from build123d import *

# Parameters (mm, degrees)
SKETCH094_W        = 71
SKETCH094_H        = 81
PAD055_DEPTH       = 5
SKETCH096_W        = 68
SKETCH096_H        = 1.5
PAD053_DEPTH       = 2
SKETCH097_W        = 64.6
SKETCH097_H        = 77.6
PAD054_DEPTH       = 2
SKETCH098_W        = 50
SKETCH098_H        = 72
POCKET086_DEPTH    = 4
SKETCH095_W        = 7.3
SKETCH095_H        = 10
PAD057_DEPTH       = 9
SKETCH099_W        = 5
SKETCH099_H        = 3.5
PAD056_DEPTH       = 9
CHAMFER028_SIZE    = 4.9
SKETCH100_R        = 2.5
POCKET087_DEPTH    = 10
SKETCH102_R        = 2.5
POCKET091_DEPTH    = 10
SKETCH101_R        = 4.5
POCKET088_DEPTH    = 3
POCKET088_FACE29_W = 64.6
POCKET088_FACE29_H = 2
POCKET089_DEPTH    = 2
POCKET089_FACE16_W = 50
POCKET089_FACE16_H = 4
PAD059_DEPTH       = 2
POCKET092_DEPTH    = 2
CHAMFER027_SIZE    = 3
CHAMFER026_SIZE    = 2
SKETCH103_W        = 50
SKETCH103_H        = 72
PAD058_DEPTH       = 2
PAD058_FACE37_W    = 0.5
PAD058_FACE37_H    = 50
POCKET090_DEPTH    = 0.5
PAD061_DEPTH       = 0.5
PAD060_DEPTH       = 0.5
POCKET093_DEPTH    = 1
CHAMFER029_SIZE    = 0.999
FILLET010_R        = 3
POCKET094_DEPTH    = 50


with BuildPart() as part:
    # Sketch094 → Pad055 (new body)
    with BuildSketch(Plane.XY):
        with Locations((-0.121221, -9.466726)):
            Rectangle(SKETCH094_W, SKETCH094_H)
    extrude(amount=-PAD055_DEPTH)

    # Sketch096 (on Face1 of Pad055) → Pad053 (join)
    with BuildSketch(Plane(origin=(0, 31.033274, 0), x_dir=(-1, 0, 0), z_dir=(0, 1, 0))):
        with Locations((0.121221, -0.75)):
            Rectangle(SKETCH096_W, SKETCH096_H)
    extrude(amount=PAD053_DEPTH)

    # Sketch097 (on Face10 of Pad053) → Pad054 (join)
    with BuildSketch(Plane.XY):
        with Locations((-0.121221, -5.766726)):
            Rectangle(SKETCH097_W, SKETCH097_H)
    extrude(amount=PAD054_DEPTH)

    # Sketch098 (on Face13 of Pad054) → Pocket086 (cut)
    with BuildSketch(Plane.XY.offset(2)):
        with Locations((-0.121221, -6.466726)):
            Rectangle(SKETCH098_W, SKETCH098_H)
    extrude(amount=-POCKET086_DEPTH, mode=Mode.SUBTRACT)

    # Sketch095 (on Face14 of Pocket086) → Pad057 (join)
    with BuildSketch(Plane.XY.offset(2)):
        with Locations((28.528779, 28.033274)):
            Rectangle(SKETCH095_W, SKETCH095_H)
        with Locations((-28.771221, 28.033274)):
            Rectangle(SKETCH095_W, SKETCH095_H)
    extrude(amount=PAD057_DEPTH)

    # Sketch099 (on Face1 of Pad057) → Pad056 (join)
    with BuildSketch(Plane.XY.offset(2)):
        with Locations((-22.621221, 31.283274)):
            Rectangle(SKETCH099_W, SKETCH099_H)
        with Locations((22.378779, 31.283274)):
            Rectangle(SKETCH099_W, SKETCH099_H)
    extrude(amount=PAD056_DEPTH)

    # Chamfer028
    chamfer028_edges = [part.edges().sort_by_distance(p)[0] for p in [
        (-20.121221, 31.283274, 11),
        (19.878779, 31.283274, 11),
    ]]
    chamfer(chamfer028_edges, length=CHAMFER028_SIZE)

    # Sketch100 (on Face12 of Chamfer028) → Pocket087 (cut)
    with BuildSketch(Plane(origin=(0, 33.033274, 0), x_dir=(-1, 0, 0), z_dir=(0, 1, 0))):
        with Locations((-28.378779, 6)):
            Circle(SKETCH100_R)
        with Locations((28.621221, 6)):
            Circle(SKETCH100_R)
    extrude(amount=-POCKET087_DEPTH, mode=Mode.SUBTRACT)

    # Sketch102 (on Face30 of Pocket087) → Pocket091 (cut)
    with BuildSketch(Plane(origin=(0, 0, -5), x_dir=(1, 0, 0), z_dir=(0, 0, -1))):
        with Locations((-28.621221, 30.966726)):
            Circle(SKETCH102_R)
        with Locations((28.378779, 30.966726)):
            Circle(SKETCH102_R)
    extrude(amount=-POCKET091_DEPTH, mode=Mode.SUBTRACT)

    # Sketch101 (on Face32 of Pocket091) → Pocket088 (cut)
    with BuildSketch(Plane(origin=(0, 0, -5), x_dir=(1, 0, 0), z_dir=(0, 0, -1))):
        with Locations((-28.621221, 30.966726)):
            Circle(SKETCH101_R)
        with Locations((28.378779, 30.966726)):
            Circle(SKETCH101_R)
    extrude(amount=-POCKET088_DEPTH, mode=Mode.SUBTRACT)

    # Pocket088 Face29 → Pocket089 (cut)
    with BuildSketch(Plane(origin=(-0.121221, -44.566726, 1), x_dir=(-1, 0, 0), z_dir=(0, -1, 0))):
        Rectangle(POCKET088_FACE29_W, POCKET088_FACE29_H)
    extrude(amount=-POCKET089_DEPTH, mode=Mode.SUBTRACT)

    # Pocket089 Face16 → Pad059 (add)
    with BuildSketch(Plane(origin=(-0.121221, -42.466726, 0), x_dir=(1, 0, 0), z_dir=(0, 1, 0))):
        Rectangle(POCKET089_FACE16_W, POCKET089_FACE16_H)
    extrude(amount=PAD059_DEPTH)

    # Pad059 Face1 → Pocket092 (cut)
    with BuildSketch(Plane(origin=(-0.121221, 29.533274, 1.353834), x_dir=(-1, 0, 0), z_dir=(0, -1, 0))):
        Polygon((-25, -9.646166), (-24.9, -9.646166), (-20, -4.746166), (-20, -0.646166), (20, -0.646166), (20, -4.746166), (24.9, -9.646166), (25, -9.646166), (25, 3.353834), (-25, 3.353834), align=None)
    extrude(amount=-POCKET092_DEPTH, mode=Mode.SUBTRACT)

    # Chamfer027
    chamfer027_edges = [part.edges().sort_by_distance(p)[0] for p in [
        (-0.121221, -49.966726, -5),
    ]]
    chamfer(chamfer027_edges, length=CHAMFER027_SIZE)

    # Chamfer026
    chamfer026_edges = [part.edges().sort_by_distance(p)[0] for p in [
        (-28.771221, 23.033274, 11),
        (28.528779, 23.033274, 11),
    ]]
    chamfer(chamfer026_edges, length=CHAMFER026_SIZE)

    # Sketch103 (on Face10 of Chamfer026) → Pad058 (join)
    with BuildSketch(Plane.XY.offset(-2)):
        with Locations((-0.121221, -4.466726)):
            Rectangle(SKETCH103_W, SKETCH103_H)
    extrude(amount=PAD058_DEPTH)

    # Pad058 Face37 → Pocket090 (cut)
    with BuildSketch(Plane(origin=(-0.121221, 31.283274, -2), x_dir=(0, -1, 0), z_dir=(0, 0, -1))):
        Rectangle(PAD058_FACE37_W, PAD058_FACE37_H)
    extrude(amount=-POCKET090_DEPTH, mode=Mode.SUBTRACT)

    # Pocket090 Face9 → Pad061 (add)
    with BuildSketch(Plane(origin=(-32.421221, 7.336396, 2.99136), x_dir=(0, 1, 0), z_dir=(-1, 0, 0))):
        Polygon((17.696878, -8.00864), (25.696878, -8.00864), (25.696878, 2.99136), (-49.903122, 2.99136), (-49.903122, 0.99136), (15.696878, 0.99136), (15.696878, -6.00864), align=None)
    extrude(amount=PAD061_DEPTH)

    # Pad061 Face19 → Pad060 (add)
    with BuildSketch(Plane(origin=(32.178779, 7.336396, 2.99136), x_dir=(0, -1, 0), z_dir=(1, 0, 0))):
        Polygon((-15.696878, -6.00864), (-15.696878, 0.99136), (49.903122, 0.99136), (49.903122, 2.99136), (-25.696878, 2.99136), (-25.696878, -8.00864), (-17.696878, -8.00864), align=None)
    extrude(amount=PAD060_DEPTH)

    # Sketch104 (on Face22 of Pad060) → Pocket093 (cut)
    with BuildSketch(Plane(origin=(0, 0, -5), x_dir=(1, 0, 0), z_dir=(0, 0, -1))):
        with BuildLine():
            ThreePointArc((-5.121221, 34), (-0.121221, 28.999784), (4.878779, 34))
            Line((-5.121221, 34), (4.878779, 34))
        make_face()
    extrude(amount=-POCKET093_DEPTH, mode=Mode.SUBTRACT)

    # Chamfer029
    chamfer029_edges = [part.edges().sort_by_distance(p)[0] for p in [
        (-0.121221, -28.999784, -5),
    ]]
    chamfer(chamfer029_edges, length=CHAMFER029_SIZE)

    # Fillet010
    fillet010_edges = [part.edges().sort_by_distance(p)[0] for p in [
        (-35.621221, -7.966726, -5),
        (35.378779, -7.966726, -5),
    ]]
    fillet(fillet010_edges, radius=FILLET010_R)

    # Sketch105 (on Face1 of Fillet010) → Pocket094 (cut)
    with BuildSketch(Plane(origin=(0, 0, -5), x_dir=(1, 0, 0), z_dir=(0, 0, -1))):
        with BuildLine():
            Line((1.378779, 37.966726), (1.378779, 49.966726))
            Line((1.378779, 49.966726), (7.378779, 49.966726))
            Line((7.378779, 49.966726), (7.378779, 37.966726))
            ThreePointArc((1.378779, 37.966726), (4.378779, 34.966726), (7.378779, 37.966726))
        make_face()
    extrude(amount=-POCKET094_DEPTH, mode=Mode.SUBTRACT)


with BuildPart() as part_1:
    # Body007 placement: moved
    add(part.part.moved(Location((0.1, -10.49, -34))))


solid = part_1.part
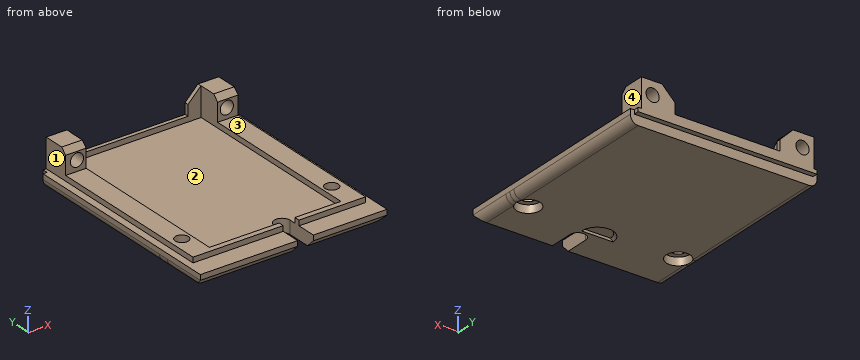
Could you check a few things on this model? Use its own coordinates, in mm. Face numbers are marked on the shaded views. A direction names the side the tool comes from. Coordinates: 2 decimals unless noted, no trailing zeros. Order: outer loops, then holes, each group sorted by start corner. A loop starts at its lowest first (then second) coordinate and runs counter-clockwise, first axis right, second up.
Q1. Suppose I cut it at A-A on y = 17.5. Please give me the cut outline in (x, z), and give its area (3 significant figures).
Q2. Suppose I cut it at B-B on x = -14. Please give me the cut outline in (y, z), and give its area (3 significant figures).
Q3. Suppose I cut it at D-D on y = -9. Please give me the cut outline in (x, z), and give its area (3 significant figures).
Q4. Will these pins go through, and if not, where does the flat tip stop? pin 1 (0.8 mm diameter, centred on x = -6, y = 21.5, fed in from +Z); pin 2 (2.5 mm diameter, centred on x = -1, y = -41, fed in from -Z); pin 3 (4 mm diameter, centred on x = -28.52, z = -28, fed in from +Y); pin 4 (5.5 mm diameter, centred on x = 31, z = -29, fed in from -Y).
Q5. Please list where these lines run through material, in increasing order: L1, parallel to Y at x = 11, z = -33; L2, parallel to Y at x = 32.5, z = -36.25; L3, parallel to Z at x = -14.5, y = -25.
Q6. Suppose I cut it at C-C on x = -29. Please give me the cut outline in (y, z).
Q7. Which directions (+Z, -Z, +X, -X, +Y, -Y) give clear straight access to the entire face, cutting with the end or side of a thin tool? Please do the marked faces 1, 2, 3 and 4.
Answer:
1. outline: (-35.52, -36) arc R3 ccw to (-32.52, -39) - (32.48, -39) arc R3 ccw to (35.48, -36) - (35.48, -34) - (32.78, -34) - (32.78, -23) - (24.98, -23) - (24.98, -34) - (-25.02, -34) - (-25.02, -23) - (-32.82, -23) - (-32.82, -34) - (-35.52, -34) - close; hole circle Ø5 at (-28.52, -28); hole circle Ø5 at (28.48, -28)
1. area: 483 mm2
2. outline: (-60.46, -36) - (-57.46, -39) - (20.54, -39) - (20.54, -35.5) - (22.54, -35.5) - (22.54, -32) - (21.04, -32) - (21.04, -34) - (-50.96, -34) - (-50.96, -32) - (-53.06, -32) - (-53.06, -34) - (-60.46, -34) - close
2. area: 411 mm2
3. outline: (-35.52, -36) arc R3 ccw to (-32.52, -39) - (32.48, -39) arc R3 ccw to (35.48, -36) - (35.48, -34) - (32.78, -34) - (32.78, -32) - (24.98, -32) - (24.98, -34) - (-25.02, -34) - (-25.02, -32) - (-32.82, -32) - (-32.82, -34) - (-35.52, -34) - close
3. area: 382 mm2
4. pin 1: stops at z = -32
4. pin 2: stops at z = -38
4. pin 3: passes through
4. pin 4: stops at y = 12.54
5. L1: y = -53.06 to -50.96, 21.04 to 22.54
5. L2: y = -60.21 to -43.48, -39.44 to 20.54
5. L3: z = -39 to -34
6. outline: (-60.46, -36) - (-57.46, -39) - (-45.93, -39) - (-45.93, -36) - (-43.91, -36) - (-43.91, -32) - (-53.06, -32) - (-53.06, -34) - (-60.46, -34) - close; (-39, -36) - (-36.98, -36) - (-36.98, -39) - (20.54, -39) - (20.54, -35.5) - (22.54, -35.5) - (22.54, -30.45) - (12.54, -30.45) - (12.54, -32) - (-39, -32) - close; (12.54, -25.55) - (22.54, -25.55) - (22.54, -23) - (14.54, -23) - (12.54, -25) - close
7. face 1: +Z, -X, +Y, -Y
7. face 2: +Z
7. face 3: +Z, +X, -X, -Y
7. face 4: +Z, +X, +Y, -Y
